Here's the drawing with two shaded views (mm, measured from the low corner). I have some questions. A direction names the side the tool comes from. Round coordinates to 2 decimals unless told otherwise and drop trailing zeros. Loops run counter-clockwise (first coordinate to the right, second up) from the corner with the lowest first, then second, coordinate; pieces in that order, holes last.
(1) If I drill on line 1 along Y through (x, z) = (88, 44); line 2 along X through (y, z) = (29, 14.5); line 3 along X through (y, z) = (66, 46), over which ranges is the centre line in solid material (lowest first)?
(2) I want a section at B-B on z = 46.5. Write out the boundary of the cut face in (x, y), plus the area to 3 significant figures.
(3) I want a section at D-D on x = 122.5. Write out the boundary of the cut face in (y, z), plus the area to 3 significant figures.
(4) Will these pins go through, and if not, where does the flat tip stop? pin 1 Ø3 at (y, z) = (81, 46.5) entering from +X; pin 2 Ø5.5 at (y, z) = (102.5, 46) entering from +X; pin 3 Ø3 at (y, z) = (12.5, 23) entering from -X.
(5) I want a section at A-A on x = 67. Write out the boundary of the cut face in (y, z), plus the area to 3 significant figures.
(6) Which directions (+Z, -Z, +X, -X, +Y, -Y) give clear straight access to the entire face, cutting with the end or side of a thin tool? Please do the marked faces 1, 2, 3 and 4.
(7) I want a section at C-C on y = 32. Write out the boundary of the cut face in (x, z), plus the area to 4 significant figures.
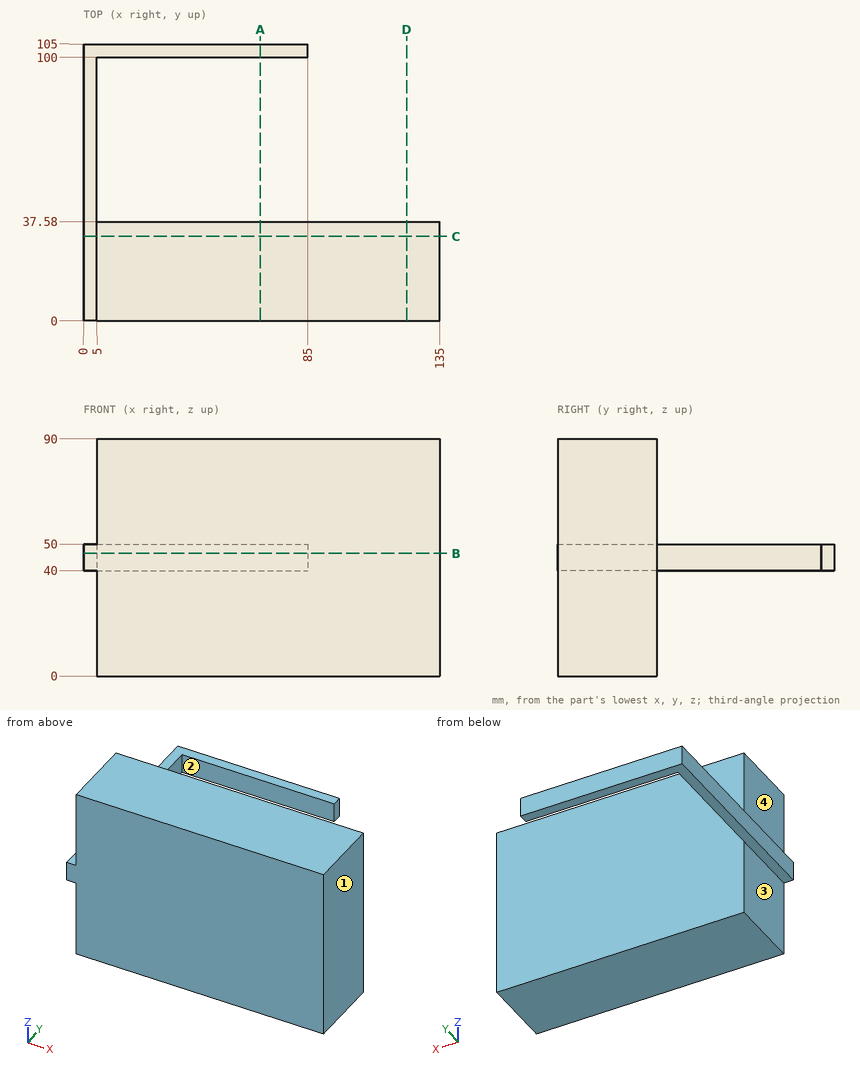
Filled sheet:
1. line 1: y = 0 to 37.58
1. line 2: x = 5 to 135
1. line 3: x = 0 to 5
2. outline: (0, 0) - (135, 0) - (135, 37.58) - (5, 37.58) - (5, 100) - (85, 100) - (85, 105) - (0, 105) - close
2. area: 5,810 mm2
3. outline: (0, 0) - (37.58, 0) - (37.58, 90) - (0, 90) - close
3. area: 3,380 mm2
4. pin 1: stops at x = 5
4. pin 2: stops at x = 85
4. pin 3: stops at x = 5
5. outline: (0, 0) - (37.58, 0) - (37.58, 90) - (0, 90) - close; (100, 40) - (105, 40) - (105, 50) - (100, 50) - close
5. area: 3,430 mm2
6. face 1: +Z, -Z, +X, +Y, -Y
6. face 2: +Z, -Z, +X
6. face 3: -Z, -X, +Y, -Y
6. face 4: +Z, -X, +Y, -Y
7. outline: (0, 40) - (5, 40) - (5, 0) - (135, 0) - (135, 90) - (5, 90) - (5, 50) - (0, 50) - close
7. area: 11,750 mm2
